Part model, mm, in its own coordinate system. A direction names the side the tool comes from. Give positions to 0.01 mm unless a question says otherwise; leave off trailing zeros. Loops run counter-clockwise (first coordinate to the right, second up) from the corner with the lowest first, then second, coordinate; pieces in that order, holes last. Notation, with made-up numbers: (14.5, 50.5) -> (53.5, 50.5) arc R15 ccw to (53.5, 59.5) -> close; hole circle Ø5 at (0.5, 9). An arc over 180 degrees is marked (long way). Write item = value, one per line.
Autodesk Inventor part; units mm, degrees
ref_plane "YZ Plane" through (0, 0, 0) normal (1, 0, 0) x (0, 1, 0)
ref_plane "XZ Plane" through (0, 0, 0) normal (0, 1, 0) x (-1, 0, 0)
ref_plane "XY Plane" through (0, 0, 0) normal (0, 0, 1) x (1, 0, 0)
sketch "Sketch1" plane through (0, 0, 0) normal (0, 1, 0) x (-1, 0, 0)
  line L0 (10.25, 4.35) -> (-10.25, 4.35)
  line L1 (-10.25, 4.35) -> (-10.25, -4.35)
  line L2 (-10.25, -4.35) -> (10.25, -4.35)
  line L3 (10.25, -4.35) -> (10.25, 4.35)
  line L4 (15.25, 26) -> (-15.25, 26)
  line L5 (-15.25, 26) -> (-15.25, -26)
  line L6 (-15.25, -26) -> (15.25, -26)
  line L7 (15.25, -26) -> (15.25, 26)
  line L8 (15.25, 26) -> (-15.25, 26)
  line L9 (-15.25, 26) -> (-15.25, 29)
  line L10 (-15.25, 29) -> (15.25, 29)
  line L11 (15.25, 29) -> (15.25, 26)
  line L12 (15.25, -26) -> (-15.25, -26)
  line L13 (-15.25, -26) -> (-15.25, -29)
  line L14 (-15.25, -29) -> (15.25, -29)
  line L15 (15.25, -29) -> (15.25, -26)
  point P0 (0, 0)
  point P1 (0, 4.35)
  point P2 (10.25, 0)
  point P3 (0, 26)
  point P4 (15.25, 0)
  dimension "d0" = 8.7
  dimension "d1" = 20.5
  dimension "d2" = 52
  dimension "d3" = 5
  dimension "d4" = 3
  dimension "d5" = 3
extrude "Extrusion1" add sketch "Sketch1" along normal blind 12
extrude "Extrusion2" add sketch "Sketch1" against normal blind 20 contours L4 L9 L10 L11 | L15 L14 L13 L6
sketch "Sketch2" plane through (0, -20, 0) normal (0, -1, 0) x (1, 0, 0)
  point P0 (0, 0)
sketch "Sketch3" plane through (-15.25, 12, 29) normal (0, 0, 1) x (1, 0, 0)
  line L0 (30.5, -32) -> (30.5, 0)
  line L1 (0, 0) -> (30.5, 0)
  line L2 (0, -32) -> (0, 0)
  line L3 (30.5, -32) -> (0, -32)
  line L4 (0, -32) -> (0, 0)
  line L5 (30.5, -32) -> (0, -32)
  line L6 (0, -32) -> (0, -28)
  line L7 (0, -28) -> (30.5, -28)
  line L8 (30.5, -28) -> (30.5, -32)
  point P0 (15.25, -12)
  dimension "d10" = 4
sketch "Sketch4" plane through (15.25, 12, -29) normal (0, 0, -1) x (-1, 0, 0)
  line L0 (30.5, -32) -> (30.5, 0)
  line L1 (0, 0) -> (30.5, 0)
  line L2 (0, -32) -> (0, 0)
  line L3 (30.5, -32) -> (0, -32)
  line L4 (30.5, -32) -> (30.5, 0)
  line L5 (0, -32) -> (30.5, -32)
  line L6 (30.5, -32) -> (30.5, -28)
  line L7 (30.5, -28) -> (0, -28)
  line L8 (0, -28) -> (0, -32)
  point P0 (15.25, -12)
  dimension "d11" = 4
extrude "Extrusion3" add sketch "Sketch4" along normal blind 20 contours L3 L2 L7 L0
extrude "Extrusion4" add sketch "Sketch3" along normal blind 20 contours L3 L2 L7 L0
shell "Shell1" thickness 3 removed faces 1 at (-3.4167, 12, -20.7833)
chamfer "Chamfer1" distance 9 angle 45 2 edges at (-12.25, 3, -16.675) (-12.25, 3, 16.675)
properties part number "servo halter"
1) Slice it at A-A, the plane x = 3.5. List the corners of the cut face in (y, z).
Resolved:
outline = (-20, -49) -> (-16, -49) -> (-16, -29) -> (12, -29) -> (12, -26) -> (3, -26) -> (3, -7.35) -> (12, -7.35) -> (12, -4.35) -> (0, -4.35) -> (0, -26) -> (-20, -26) -> close; (-20, 26) -> (0, 26) -> (0, 4.35) -> (12, 4.35) -> (12, 7.35) -> (3, 7.35) -> (3, 26) -> (12, 26) -> (12, 29) -> (-16, 29) -> (-16, 49) -> (-20, 49) -> close
2) Drill centre lines: line 1 along Z through (x, y) = (12, 6); line 2 along Z through (x, y) = (-4.5, 6); line 3 along Z through (x, y) = (4, -14.5). Where is each one in solid material? Low to high. Write a range as [from, to].
Resolved:
line_1 = [-29, -26], [-7.35, 7.35], [26, 29]
line_2 = [-29, -26], [-7.35, -4.35], [4.35, 7.35], [26, 29]
line_3 = [-29, -26], [26, 29]
3) Which spindle directions (+Z, -Z, +X, -X, +Y, -Y) get a long thin tool onto all of the face, cutting with end or side? Do faces 4 (the face through (3, 7, -7.35)), 5 (the face through (0, -2, -29)), 6 (the face through (0, 0, 6)), 7 (the face through (0, -20, 37)), 8 (the face through (-10.25, 6, 0)). Say none if no direction does.
Resolved:
face_4 = +Y
face_5 = -Z, +X, -X, +Y
face_6 = +X, -X, -Y
face_7 = +Z, -Z, +X, -X, -Y
face_8 = +Y, -Y
4) Pull direction Z, two halves, no side cores. Call faces 1 (the face through (0, -18, 49)), 2 (the face through (0, -20, -37)), 3 (the face through (3, 7, -26)): pulls with the +Z half, pulls with the -Z half, needs draft (parallel to the pull), parting line crosses it, or undercut.
Resolved:
face_1 = pulls with the +Z half
face_2 = needs draft
face_3 = undercut
5) Slice it at D-D, the plane y = 9. List the corners of the cut face in (x, z).
Resolved:
outline = (-15.25, -29) -> (15.25, -29) -> (15.25, 29) -> (-15.25, 29) -> close; hole (-10.25, -4.35) -> (10.25, -4.35) -> (10.25, 4.35) -> (-10.25, 4.35) -> close; hole (-9.25, -26) -> (12.25, -26) -> (12.25, -7.35) -> (-9.25, -7.35) -> close; hole (-9.25, 7.35) -> (12.25, 7.35) -> (12.25, 26) -> (-9.25, 26) -> close
6) Slice it at B-B, the plane y = -8. List the corners of the cut face in (x, z).
Resolved:
outline = (-15.25, -29) -> (15.25, -29) -> (15.25, -26) -> (-15.25, -26) -> close; (-15.25, 26) -> (15.25, 26) -> (15.25, 29) -> (-15.25, 29) -> close
7) Drop flat-ended pins along their axis: P1, Ø8, axis at x = 11, y = -11, coming from the +Z side; P2, Ø10, axis at x = 2.5, y = -9, coming from the -Z side; P3, Ø12.5, axis at x = 3.5, z = -15, coming from the +Y side; P4, Ø1.5, axis at y = 6, z = -30, coming from the +X side. Give the stop position or say it passes through.
Resolved:
P1 = 29
P2 = -29
P3 = 3
P4 = through
